Work out the finished part from the listing and answer in its coordinate system (mm). Face numbers are marked on the shaded views. A direction names the side the tool comes from. Round coordinates to 2 decimals unless told otherwise and drop trailing zeros. Loops run counter-clockwise (first coordinate to the right, second up) from the corner with the lowest first, then second, coordinate; pieces in that order, holes last.
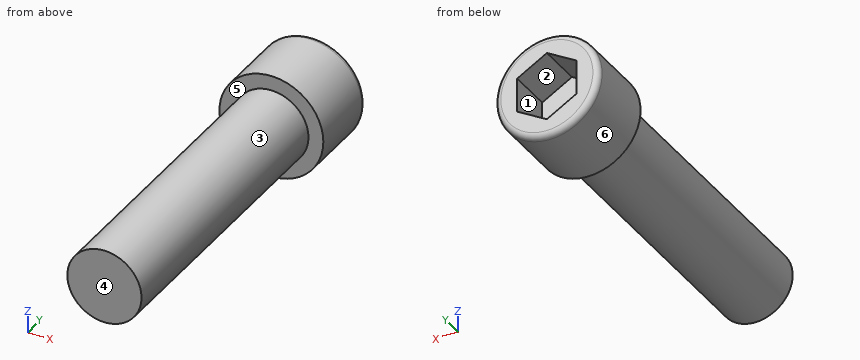
```python
from build123d import *

# Parameters (mm, degrees)
SKETCH1_R           = 1.75
BOSS_EXTRUDE1_DEPTH = 2.5
SKETCH3_R           = 1.25
BOSS_EXTRUDE2_DEPTH = 10
FILLET1_R           = 0.2
CUT_EXTRUDE1_DEPTH  = 1.5


with BuildPart() as part:
    # Sketch1 → Boss-Extrude1 (new body)
    with BuildSketch(Plane(origin=(0, 0, 0), x_dir=(1, 0, 0), z_dir=(0, 1, 0))):
        Circle(SKETCH1_R)
    extrude(amount=BOSS_EXTRUDE1_DEPTH)

    # Sketch3 → Boss-Extrude2 (add)
    with BuildSketch(Plane.XZ):
        Circle(SKETCH3_R)
    extrude(amount=BOSS_EXTRUDE2_DEPTH)

    # Fillet1
    fillet1_edges = [part.edges().sort_by_distance(p)[0] for p in [
        (-1.75, 2.5, 0),
    ]]
    fillet(fillet1_edges, radius=FILLET1_R)

    # Sketch4 → Cut-Extrude1 (cut)
    with BuildSketch(Plane(origin=(0, 2.5, 0), x_dir=(1, 0, 0), z_dir=(0, 1, 0))):
        Polygon((0, -1.154700538), (1, -0.577350269), (1, 0.577350269), (0, 1.154700538), (-1, 0.577350269), (-1, -0.577350269), align=None)
    extrude(amount=-CUT_EXTRUDE1_DEPTH, mode=Mode.SUBTRACT)


solid = part.part
```
1. Given pin 1 (1.5 mm diameter, centred on x = 1, y = -7.5, fed in from +Z); pin 2 (1 mm diameter, centred on x = -1, y = -4, fed in from -Z), each flat-ended and moving along its own axis, determine where each tip first touches the part or whether it passes through.
Answer key:
pin 1: stops at z = 1.22
pin 2: stops at z = -1.15
2. Find section B-B (y = -2.5). Write down the section's boundary in (x, z), then the cut area to 3 significant figures.
Answer key:
outline: circle Ø2.5 at (0, 0)
area: 4.91 mm2
3. Which of the six approach directions +Z, -Z, +X, -X, +Y, -Y give full straight-line access (tool end or side, diameter ignored) to the marked faces 5 and 6?
Answer key:
face 5: -Y
face 6: +Y, -Y
4. Find section A-A (z = 0). Write down the section's boundary in (x, y), then the cut area to 3 significant figures.
Answer key:
outline: (-1.75, 0) - (-1.25, 0) - (-1.25, -10) - (1.25, -10) - (1.25, 0) - (1.75, 0) - (1.75, 2.3) arc R0.2 ccw to (1.55, 2.5) - (1, 2.5) - (1, 1) - (-1, 1) - (-1, 2.5) - (-1.55, 2.5) arc R0.2 ccw to (-1.75, 2.3) - close
area: 30.7 mm2
5. Consider probe 1 along Y at (x, z) = (-0.1, -1.4); probe 2 along Y at (x, z) = (0.3, -0.25); probe 3 along X at (y, z) = (-7.5, -0.35). Determine where each line is inside the solid, lowest interval first.
Answer key:
probe 1: y = 0 to 2.5
probe 2: y = -10 to 1
probe 3: x = -1.2 to 1.2
6. Determine the mould class of the marked faces 1, 2, 3 and 4 for opening direction Z: +Z half, -Z half, draft (parallel to the pull), parting line (faces both ways), or undercut.
Answer key:
face 1: undercut
face 2: undercut
face 3: parting line
face 4: draft
7. Find section C-C (y = 0.25). Write down the section's boundary in (x, z).
Answer key:
outline: circle Ø3.5 at (0, 0)
